Can you work these out from the drawing? Everything is in mm from the part's minimum corner. A direction names the side the tool comes from. Give positions to 0.01 mm unless a question says otherwise; leave off trailing zeros. Loops run counter-clockwise (first coordinate to the right, second up) from the corner with the lowest first, then second, coordinate; pieces in that order, holes last. Notation, with made-up numbers: (-23, 58.5) - (-7, 58.5) arc R18 cw to (-7, 72.5) - close; hole circle Ø5 at (57, 42). An arc over 180 degrees is marked (long way). Write each question's results on one line, items separated by ' | '. Start each with the question number.
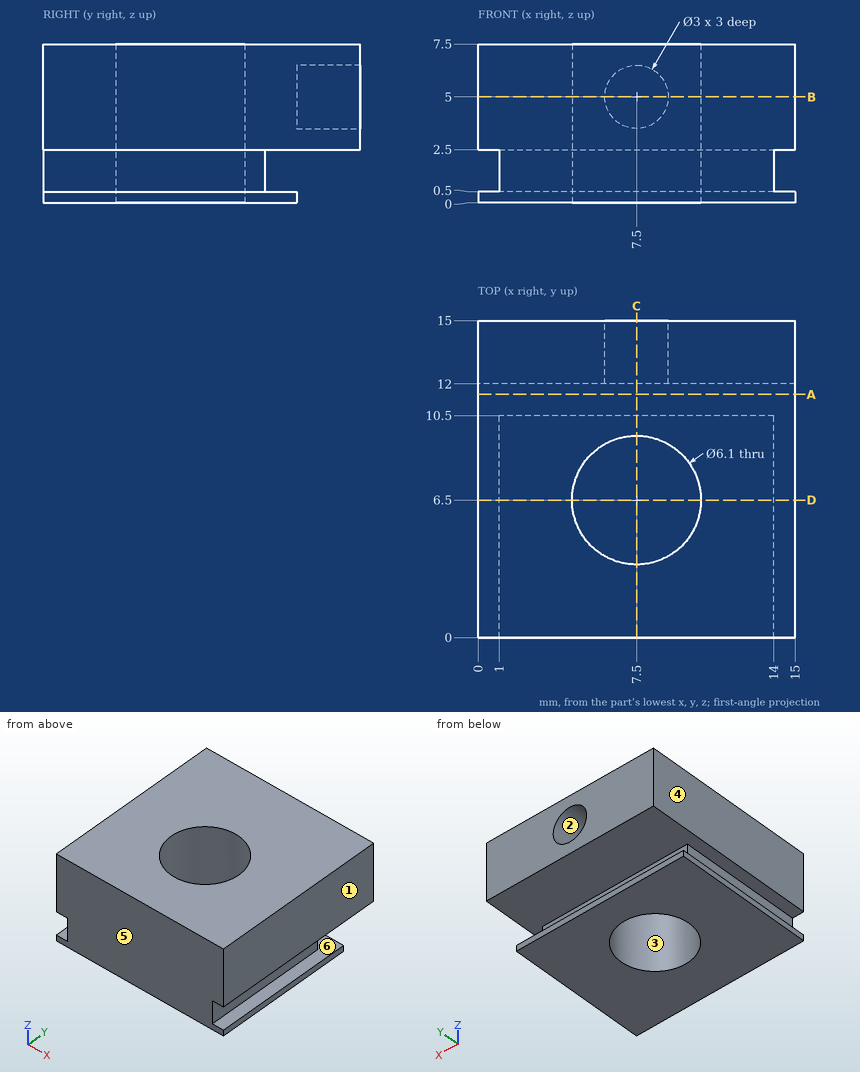
Q1. If we mould it in two halves opening along X, with no side actions, what happens to the marked faces 1, 2, 3 and 4? For each: +X half, -X half, draft (parallel to the pull), parting line (faces both ways), or undercut.
Q2. I want a section at A-A, the plane y = 11.5. List the corners of the cut face in (x, z) for me, then the cut area to 3 significant figures.
Q3. Which directions (+Z, -Z, +X, -X, +Y, -Y) give clear straight access to the entire face, cutting with the end or side of a thin tool? Please do the marked faces 5 and 6.
Q4. I want a section at B-B, the plane z = 5. List the corners of the cut face in (x, y) for me, then the cut area to 3 significant figures.
Q5. I need wall thicknesses on L1, parallel to Z at x = 4, y = 11; L2, parallel to Z at x = 5, y = 14; L3, parallel to X at y = 3.75, z = 0.75. Which ranges of each line are inside material? Lowest first, please. Write a range as from..to.
Q6. I'm going to push flat-ended pins straight in: pin 1 Ø0.6 at (x, z) = (5, 1.5) entering from +Y; pin 2 Ø0.6 at (x, z) = (10, 0) entering from +Y. Where does each tip first touch, or does it pass through?
Q7. I want a section at D-D, the plane y = 6.5. List the corners of the cut face in (x, z) for me.
Q8. I want a section at C-C, the plane x = 7.5. List the corners of the cut face in (y, z) for me.
Conclusion:
1) face 1: +X half | face 2: undercut | face 3: undercut | face 4: -X half
2) outline: (0, 0) - (15, 0) - (15, 0.5) - (0, 0.5) - close; (0, 2.5) - (15, 2.5) - (15, 7.5) - (0, 7.5) - close | area: 82.5 mm^2
3) face 5: +Z, -Z, +X, -X, -Y | face 6: +Y
4) outline: (0, 0) - (15, 0) - (15, 15) - (9, 15) - (9, 12) - (6, 12) - (6, 15) - (0, 15) - close; hole circle Ø6.1 at (7.5, 6.5) | area: 187 mm^2
5) L1: 0..0.5, 2.5..7.5 | L2: 2.5..7.5 | L3: 1..6.18, 8.82..14
6) pin 1: y = 10.5 | pin 2: y = 12
7) outline: (0, 0) - (4.45, 0) - (4.45, 7.5) - (0, 7.5) - (0, 2.5) - (1, 2.5) - (1, 0.5) - (0, 0.5) - close; (10.55, 0) - (15, 0) - (15, 0.5) - (14, 0.5) - (14, 2.5) - (15, 2.5) - (15, 7.5) - (10.55, 7.5) - close
8) outline: (0, 0) - (3.45, 0) - (3.45, 7.5) - (0, 7.5) - close; (9.55, 0) - (12, 0) - (12, 0.5) - (10.5, 0.5) - (10.5, 2.5) - (15, 2.5) - (15, 3.5) - (12, 3.5) - (12, 6.5) - (15, 6.5) - (15, 7.5) - (9.55, 7.5) - close
